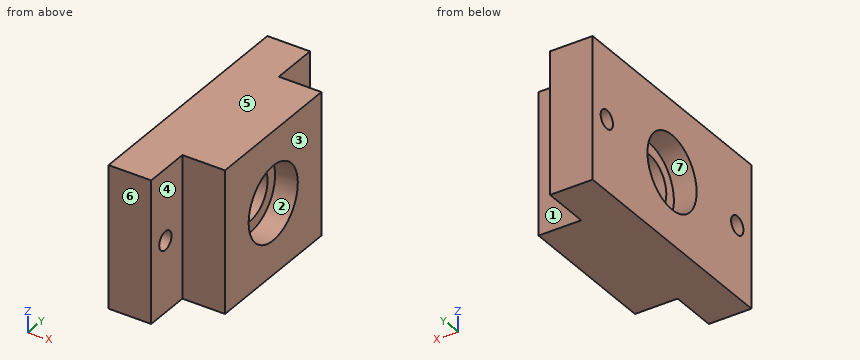
```python
from build123d import *

# Parameters (mm, degrees)
BOSS_EXTRUDE1_DEPTH        = 50
F_6_5_6_5_DIAMETER_HOLE1_D = 6.5


with BuildPart() as part:
    # Sketch1 → Boss-Extrude1 (new body)
    with BuildSketch(Plane.XY):
        Polygon((0, 42), (0, -42), (15, -42), (15, -25.5), (30, -25.5), (30, 25.5), (15, 25.5), (15, 42), align=None)
    extrude(amount=BOSS_EXTRUDE1_DEPTH)

    # Ø6.5 (6.5) Diameter Hole1 (through all)
    with Locations(Plane(origin=(15, 0, 0), x_dir=(0, 0, -1), z_dir=(1, 0, 0))):
        with Locations((-25, -34.5), (-25, 34.5)):
            Hole(F_6_5_6_5_DIAMETER_HOLE1_D / 2)

    # Sketch4 → Cut-Revolve1 (revolve, cut)
    with BuildSketch(Plane(origin=(0, 0, 0), x_dir=(1, 0, 0), z_dir=(0, 1, 0))):
        Polygon((0, -25), (0, -38), (8, -38), (8, -34), (22, -34), (22, -38), (30, -38), (30, -25), align=None)
    revolve(axis=Axis((0, 0, 25), (1, 0, 0)), mode=Mode.SUBTRACT)


solid = part.part
```
Geometry: final body of the model. Coordinates: model frame, mm. Face numbers are marked on the shaded views. A direction names the side the tool comes from. Round coordinates to 2 decimals unless told otherwise and drop trailing zeros. Write each loop counter-clockwise with the first axis right and the second up, starting at its lowest first coordinate (ties: lowest second). Pieces come first, ordered by that corner, then holes. Notation, with made-up numbers: M 13,46 L 37,46 A23 cw 37,77 Z; hole C 43,45 d2. An arc over 180 degrees is marked long. Answer in a Markdown table with one row per item. Add a question column.
(1) Draft query along Z for the marked faces 5, 6 and 7. Return one class per face: pulls with the +Z half, pulls with the -Z half, needs draft (parallel to the pull), parting line crosses it, or undercut.
(2) Cut plane B-B, the plane z = 25. Return the cut outline in (x, y), then the cut area to 3 significant figures.
(3) Contact query for flat-ended pins moving along their axis: pin 1 (7.5 mm diameter, centred on x = 24.5, z = 26, fed in from +Y); pin 2 (5 mm diameter, centred on y = -34.5, z = 13, fed in from +X); pin 3 (1 mm diameter, centred on x = 24, z = 7.5, fed in from -Y). Output: stop coordinate, or through.
(4) Ray query, L1, parallel to Y at x = 3.5, z = 25; L2, parallel to Z at x = 24.25, y = 0; L3, parallel to Z at x = 14.5, y = 0. Return the intervals inside material, ascending.
(5) Reachability of the marked faces 1, 2, 3 and 4 from +Z, -Z, +X, -X, +Y, -Y: full face, straight path, thin tool, end or side. Return the list, or none.
(6) Cut plane D-D, the plane z = 7. Return the cut outline in (x, y), then the cut area to 4 significant figures.
(7) Cut plane A-A, the plane y = 34.5. Return the cut outline in (x, z).
(8) Cut plane C-C, the plane x = 6.75. Return the cut outline in (y, z), then the cut area to 3 significant figures.
Established:
| question | item | result |
|---|---|---|
| 1 | face 5 | pulls with the +Z half |
| 1 | face 6 | needs draft |
| 1 | face 7 | undercut |
| 2 | outline | M 0,-42 L 15,-42 L 15,-37.75 L 0,-37.75 Z; M 0,-31.25 L 15,-31.25 L 15,-25.5 L 30,-25.5 L 30,-13 L 22,-13 L 22,-9 L 8,-9 L 8,-13 L 0,-13 Z; M 0,13 L 8,13 L 8,9 L 22,9 L 22,13 L 30,13 L 30,25.5 L 15,25.5 L 15,31.25 L 0,31.25 Z; M 0,37.75 L 15,37.75 L 15,42 L 0,42 Z |
| 2 | area | 1,160 mm² |
| 3 | pin 1 | y = 25.5 |
| 3 | pin 2 | x = 15 |
| 3 | pin 3 | y = -25.5 |
| 4 | L1 | -42 to -37.75, -31.25 to -13, 13 to 31.25, 37.75 to 42 |
| 4 | L2 | 0 to 12, 38 to 50 |
| 4 | L3 | 0 to 16, 34 to 50 |
| 5 | face 1 | +Z, -Z, +X, +Y |
| 5 | face 2 | +X |
| 5 | face 3 | +Z, -Z, +X, +Y, -Y |
| 5 | face 4 | +Z, -Z, +X, -Y |
| 6 | outline | M 0,-42 L 15,-42 L 15,-25.5 L 30,-25.5 L 30,25.5 L 15,25.5 L 15,42 L 0,42 Z |
| 6 | area | 2,025 mm² |
| 7 | outline | M 0,0 L 15,0 L 15,21.75 L 0,21.75 Z; M 0,28.25 L 15,28.25 L 15,50 L 0,50 Z |
| 8 | outline | M -42,0 L 42,0 L 42,50 L -42,50 Z; hole C -34.5,25 d6.5; hole C 0,25 d26; hole C 34.5,25 d6.5 |
| 8 | area | 3,600 mm² |
